```python
from build123d import *

# Parameters (mm, degrees)
F1_DEPTH  = 41.91
F2_R      = 9.525
F3_DEPTH  = 38.1
F6_DEPTH  = 41.91
F7_R      = 72.9800133434
F8_R      = 6.35
F4_R      = 1.5875
F9_DEPTH  = 128.27
F10_DEPTH = 90.678
F11_R     = 5.08
F13_DEPTH = 39.624


with BuildPart() as f1:
    # F0 (on Front) → F1 (new body)
    with BuildSketch(Plane.XZ):
        Polygon((0, 62.717492425), (0, 0), (301.1213292729, 0), (301.1213292729, 19.05), align=None)
    extrude(amount=-F1_DEPTH)

    # F2 (on face) → F3 (cut)
    with BuildSketch(Plane(origin=(0, 0, 0), x_dir=(0, -1, 0), z_dir=(-1, 0, 0))):
        with Locations((-20.955, 33.02)):
            Circle(F2_R)
    extrude(amount=-F3_DEPTH, mode=Mode.SUBTRACT)

    # F5 (on face) → F6 (cut)
    with BuildSketch(Plane.XZ):
        Polygon((36.6667471826, 54.8031888902), (68.9622256454, 4.6046015509), (253.1122256454, 4.6046015509), (270.404113194, 23.2097251733), (298.0381529682, 19.0862017092), (298.0381529682, 0), (301.1213292729, 0), (301.1213292729, 19.05), (0, 62.717492425), (0, 54.8031888902), align=None)
    extrude(amount=-F6_DEPTH, mode=Mode.SUBTRACT)

    # F7
    f7_edges = [f1.edges().sort_by_distance(p)[0] for p in [
        (68.962226, 20.955, 4.604602),
    ]]
    fillet(f7_edges, radius=F7_R)

    # F8
    f8_edges = [f1.edges().sort_by_distance(p)[0] for p in [
        (36.666747, 20.955, 54.803189),
        (0, 20.955, 54.803189),
    ]]
    fillet(f8_edges, radius=F8_R)

    # F4 (on face) → F9 (cut)
    with BuildSketch(Plane.XZ):
        with Locations((279.8462808132, 9.525)):
            Circle(F4_R)
    extrude(amount=-F9_DEPTH, mode=Mode.SUBTRACT)

    # F4 (on face) → F10 (cut)
    with BuildSketch(Plane.XZ):
        with Locations((279.8462808132, 9.525)):
            Circle(F4_R)
        with Locations((25.7700905204, 9.525)):
            Circle(F4_R)
    extrude(amount=-F10_DEPTH, mode=Mode.SUBTRACT)

    # F11
    f11_edges = [f1.edges().sort_by_distance(p)[0] for p in [
        (298.038153, 20.955, 19.086202),
        (270.404113, 20.955, 23.209725),
        (284.221133, 41.91, 21.147963),
        (284.221133, 0, 21.147963),
        (298.038153, 20.955, 0),
    ]]
    fillet(f11_edges, radius=F11_R)

    # F12 (on face) → F13 (cut)
    with BuildSketch(Plane.XY.offset(4.6046015509)):
        Polygon((108.789094354, 0), (226.7754729672, 0), (205.8822836606, 5.4408400638), (129.6822836606, 5.4408400638), align=None)
        Polygon((205.8822836606, 36.4691599362), (226.7754729672, 41.91), (108.789094354, 41.91), (129.6822836606, 36.4691599362), align=None)
    extrude(amount=-F13_DEPTH, mode=Mode.SUBTRACT)


solid = f1.part
```
Build history of the part. All positions in model axes, mm. A direction names the side the tool comes from. Round coordinates to 2 decimals unless told otherwise and drop trailing zeros. Loops run counter-clockwise (first coordinate to the right, second up) from the corner with the lowest first, then second, coordinate; pieces in that order, holes last.
Item 1: Saw through at C-C (x = 245). List the corners of the cut face in (y, z), then the cut area to 3 significant figures.
Item 2: Which spindle directions (+Z, -Z, +X, -X, +Y, -Y) get a long thin tool onto all of the face, cutting with end or side? Do faces 1 (the face through (119.38, 2.76, 2.33)), 2 (the face through (283.2, 20.7, 21.3)), 3 (the face through (167, 36.469, 2)), 4 (the face through (29, 0, 22)), 5 (the face through (260.74, 20.66, 12.81)). Say none if no direction does.
Item 3: Saw through at A-A (y = 21.5). State how many separate pieces and enclosed holes the cut face has, then the cut area to 3 significant figures.
Item 4: Pin check, flat tips, straight feed: P1, Ø4, axis at x = 255.5, y = 33, coming from the +Z side; P2, Ø2, axis at y = 35, z = 34.5, coming from the +X side; P3, Ø3.5, axis at x = 153, z = 2.5, coming from the -Y side. Stop position of each tip, or through.
Item 5: Two-plate mould, pull along X, no slides. Class faces 6 (the face through (119.089, 39.228, 2.335)), 7 (the face through (0, 21, 19)), 8 (the face through (36.282, 21.248, 54.006)): released by +X, released by -X, zero draft, split by the parting line, or undercut.
Item 6: Drill centre lines: line 1 along Z through (x, y) = (118.5, 12.5); line 2 along X through (y, z) = (15.5, 11.5); line 3 along Y through (x, z) = (142, 3). Where is each one in solid material? Low to high.
Item 7: Saw through at B-B (z = 33.02). List the corners of the cut face in (x, y), then the cut area to 3 significant figures.
Item 8: Saw through at D-D (x = 181.5). List the corners of the cut face in (y, z), then the cut area to 3 significant figures.
Worked answers:
1. outline: (0, 0) - (41.91, 0) - (41.91, 4.6) - (0, 4.6) - close
1. area: 193 mm2
2. face 1: +Z, -Z, -Y
2. face 2: +Z, +X, +Y, -Y
2. face 3: +Z, -Z, +Y
2. face 4: +Z, -Z, +X, -X, -Y
2. face 5: +Z, +Y, -Y
3. separate pieces: 1
3. enclosed holes: 2
3. area: 4,130 mm2
4. P1: stops at z = 9.33
4. P2: stops at x = 50.63
4. P3: stops at y = 5.44
5. face 6: undercut
5. face 7: released by -X
5. face 8: released by +X
6. line 1: z = 0 to 4.6
6. line 2: x = 0 to 77.82, 259.52 to 298.04
6. line 3: y = 5.44 to 36.47
7. outline: (0, 0) - (51, 0) - (51, 41.91) - (0, 41.91) - (0, 30.48) - (38.1, 30.48) - (38.1, 11.43) - (0, 11.43) - close
7. area: 1,410 mm2
8. outline: (5.44, 0) - (36.47, 0) - (36.47, 4.6) - (5.44, 4.6) - close
8. area: 143 mm2
